Can you work these out from the model? Positions are in its coordinate system, mm. Coordinates: 2 decimals unless noted, no trailing zeros. Order: outer loops, then holes, each group sorted by start corner. A loop starts at its lowest first (then second) coordinate and runs counter-clockwise, first axis right, second up. Notation, with made-up numbers: (-13.5, -31) -> (25.5, -31) arc R20 cw to (25.5, 0) -> close; hole circle Ø2 at (-21.5, 15). An arc over 180 degrees is marked (long way). Return JSON: item names as keys, results as strings. Group by question number.
1) If we section it at D-D, the plane x = 173.5: Please give me the cut outline in (y, z).
2) For pin 1 (6 mm diameter, centred on x = 115.5, y = 11.5, fed in from -Z); pin 2 (6 mm diameter, centred on x = 65.5, y = 11, fed in from +Z); pin 3 (1.8 mm diameter, centred on x = 36.5, z = 20, fed in from +Y), each with a flat end and sliding along its axis, tell me the tip position at first contact or that it passes through.
3) If we section it at B-B, the plane y = 9.5: State how many separate pieces and enclosed holes the cut face has, then the cut area to 3 significant figures.
4) If I drill on probe 1 along Z at (x, y) = (42, 9); probe 2 along X at (y, z) = (4.75, 10) (3 decimals); probe 3 along X at (y, z) = (1.8, 0) (3 decimals), over which ranges is the centre line in solid material (lowest first)? Write a range as from..to.
5) If we section it at A-A, the plane x = 132: Please give me the cut outline in (y, z), then the cut area to 3 significant figures.
6) If we section it at C-C, the plane z = 37.5: Please give me the cut outline in (x, y) (3 decimals), then the cut area to 3 significant figures.
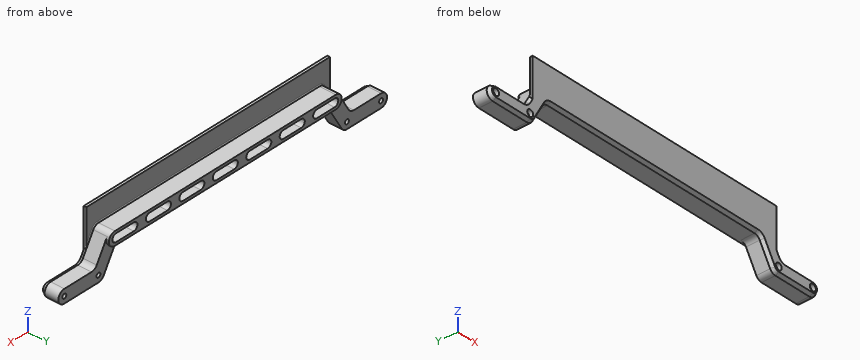
from build123d import *

# Parameters (mm, degrees)
SKETCH_1_R                 = 1.65
EXTRUDE_1_DEPTH            = 15
FILLET_1_R                 = 5
CHAMFER_1_SIZE             = 1.5
CHAMFER_1_SIZE2            = 2.598076211
SKETCH_3_R                 = 2.5
CUT_EXTRUDE_1_DEPTH        = 3
SKETCH_4_W                 = 353.760068279
SKETCH_4_H                 = 71.916373997
CUT_EXTRUDE_2_DEPTH        = 2
FILLET_2_R                 = 5
CUT_EXTRUDE_3_DEPTH        = 12
PATTERN_LINEAR_1_COUNT     = 4
PATTERN_LINEAR_1_PITCH     = 28
PATTERN_LINEAR_1_COL_COUNT = 4
PATTERN_LINEAR_1_COL_PITCH = 28
EXTRUDE_2_DEPTH            = 2
FILLET_3_R                 = 1


# Some blends are built 0.0001 mm under size
with BuildPart() as part:
    # 草图1 → 凸台-拉伸1 (new body)
    with BuildSketch(Plane(origin=(0, 0, 0), x_dir=(1, 0, 0), z_dir=(0, 1, 0))):
        with BuildLine():
            Line((14.275, 5), (-14.275, 5))
            ThreePointArc((-14.275, 5), (-19.275, 0), (-14.275, -5))
            Line((-14.275, -5), (11.388248654, -5))
            Line((11.388248654, -5), (21.491878365, -22.5))
            ThreePointArc((21.491878365, -22.5), (23.322005384, -24.330127019), (25.822005384, -25))
            Line((25.822005384, -25), (210.627994616, -25))
            ThreePointArc((210.627994616, -25), (213.127994616, -24.330127019), (214.958121635, -22.5))
            Line((214.958121635, -22.5), (225.061751346, -5))
            Line((225.061751346, -5), (250.725, -5))
            ThreePointArc((250.725, -5), (255.725, 0), (250.725, 5))
            Line((250.725, 5), (222.175, 5))
            ThreePointArc((222.175, 5), (219.675, 4.330127019), (217.844872981, 2.5))
            Line((217.844872981, 2.5), (207.74124327, -15))
            Line((207.74124327, -15), (28.70875673, -15))
            Line((28.70875673, -15), (18.605127019, 2.5))
            ThreePointArc((18.605127019, 2.5), (16.775, 4.330127019), (14.275, 5))
        make_face()
        with Locations(Location((-14.275, 0, 0), (0, 0, 270))):
            Circle(SKETCH_1_R, mode=Mode.SUBTRACT)
        with Locations(Location((14.275, 0, 0), (0, 0, 270))):
            Circle(SKETCH_1_R, mode=Mode.SUBTRACT)
        with Locations(Location((222.175, 0, 0), (0, 0, 270))):
            Circle(SKETCH_1_R, mode=Mode.SUBTRACT)
        with Locations(Location((250.725, 0, 0), (0, 0, 270))):
            Circle(SKETCH_1_R, mode=Mode.SUBTRACT)
    extrude(amount=EXTRUDE_1_DEPTH)

    # 圆角1
    fillet_1_edges = [part.edges().sort_by_distance(p)[0] for p in [
        (225.061751346, 7.5, 5),
        (11.388248654, 7.5, 5),
        (28.70875673, 7.5, 15),
        (207.74124327, 7.5, 15),
    ]]
    fillet(fillet_1_edges, radius=FILLET_1_R)

    # 倒角1
    chamfer_1_edges = [part.edges().sort_by_distance(p)[0] for p in [
        (255.725, 0, 0),
        (219.288248654, 0, 15),
        (213.127994616, 0, 24.330127019),
        (118.225, 0, 25),
        (23.322005384, 0, 24.330127019),
        (-2.886751346, 0, 5),
        (-19.275, 0, 0),
        (0, 0, -5),
        (16.775, 0, -4.330127019),
        (22.935254038, 0, 5),
        (219.675, 0, -4.330127019),
        (236.45, 0, -5),
        (118.225, 0, 15),
        (213.514745962, 0, 5),
        (239.336751346, 0, 5),
        (17.161751346, 0, 15),
        (207.354491924, 0, 14.330127019),
        (29.095508076, 0, 14.330127019),
        (225.448502692, 0, 5.669872981),
        (11.001497308, 0, 5.669872981),
    ]]
    chamfer_1_side = [part.faces().sort_by_distance(p)[0] for p in [
        (216.892549382, 0, 13.616842381),
    ]]
    chamfer(chamfer_1_edges, length=CHAMFER_1_SIZE, length2=CHAMFER_1_SIZE2, reference=chamfer_1_side[0])

    # 草图3 → 切除-拉伸1 (cut)
    with BuildSketch(Plane(origin=(0, 0, 0), x_dir=(1, 0, 0), z_dir=(0, 1, 0))):
        with Locations(Location((-14.275, 0, 0), (0, 0, 270))):
            Circle(SKETCH_3_R)
        with Locations(Location((14.275, 0, 0), (0, 0, 270))):
            Circle(SKETCH_3_R)
        with Locations(Location((250.725, 0, 0), (0, 0, 270))):
            Circle(SKETCH_3_R)
        with Locations(Location((222.175, 0, 0), (0, 0, 270))):
            Circle(SKETCH_3_R)
    extrude(amount=CUT_EXTRUDE_1_DEPTH, mode=Mode.SUBTRACT)

    # 草图4 → 切除-拉伸2 (cut)
    with BuildSketch(Plane(origin=(0, 15, 0), x_dir=(1, 0, 0), z_dir=(0, 1, 0))):
        with Locations((127.300161481, 20.958186999)):
            Rectangle(SKETCH_4_W, SKETCH_4_H)
    extrude(amount=-CUT_EXTRUDE_2_DEPTH, mode=Mode.SUBTRACT)

    # 圆角2
    fillet_2_edges = [part.edges().sort_by_distance(p)[0] for p in [
        (17.161751346, 14, 15),
        (219.288248654, 14, 15),
    ]]
    fillet(fillet_2_edges, radius=FILLET_2_R - 0.0001)  # a hair under: the kernel refuses the full size

    # 草图5 → 切除-拉伸3 (cut)
    with BuildSketch(Plane(origin=(0, 15, 0), x_dir=(1, 0, 0), z_dir=(0, 1, 0))):
        with BuildLine():
            Line((110.725, -17), (125.725, -17))
            ThreePointArc((125.725, -17), (128.725, -20), (125.725, -23))
            Line((125.725, -23), (110.725, -23))
            ThreePointArc((110.725, -23), (107.725, -20), (110.725, -17))
        make_face()
    cut_extrude_3 = extrude(amount=-CUT_EXTRUDE_3_DEPTH, mode=Mode.SUBTRACT)

    # 阵列(线性)1: 切除-拉伸3 ×4
    with Locations(*[(i * PATTERN_LINEAR_1_PITCH, 0, 0) for i in range(1, PATTERN_LINEAR_1_COUNT)]):
        add(cut_extrude_3, mode=Mode.SUBTRACT)

    # 阵列(线性)1 col: 切除-拉伸3 ×4
    with Locations(*[(-i * PATTERN_LINEAR_1_COL_PITCH, 0, 0) for i in range(1, PATTERN_LINEAR_1_COL_COUNT)]):
        add(cut_extrude_3, mode=Mode.SUBTRACT)

    # 草图6 → 凸台-拉伸2 (add)
    with BuildSketch(Plane.XZ):
        Polygon((25.533330249, 23.5), (210.339319482, 23.5), (220.175, 6.464101615), (220.175, 23.5), (220.175, 40), (16.275, 40), (16.275, 23), (16.275, 7.464101615), align=None)
    extrude(amount=-EXTRUDE_2_DEPTH)

    # 圆角3
    # the kernel refuses this fillet: 1 mm, written as the material it adds along each edge
    with BuildSketch(Plane(origin=(214.659083529, 2, 22.327350269), x_dir=(0.4330127018948014, 0.8660254037827173, 0.2500000000014904), z_dir=(0.4999999999999995, 0, -0.866025403784439))) as fillet_3_piece_1_section:
        with BuildLine():
            CenterArc((1.496511696, 0.592034292), FILLET_3_R, 150, 66.301500994)
            Line((0.630486292, 1.092034292), (0.613165784, 1.102034292))
            Line((0.613165784, 1.102034292), (-0.017320508, 0.01))
            Line((-0.017320508, 0.01), (0, -0.02))
            ThreePointArc((0, -0.02), (0.345299462, -0.02), (0.674480668, -0.011840686))
            Line((0.674480668, -0.011840686), (0.690598923, 0))
        make_face()
    fillet_3_piece_1 = extrude(amount=14.184264403, mode=Mode.PRIVATE)
    fillet_3_piece_1 = split(fillet_3_piece_1, bisect_by=Plane(origin=(220.175, 2.148183279, 18.272519996), z_dir=(-1, 0, 0)), keep=Keep.TOP, mode=Mode.PRIVATE)
    add(fillet_3_piece_1)
    with BuildSketch(Plane(origin=(210.627994616, 2, 20), x_dir=(0, 0, 1), z_dir=(-1, 0, 0))) as fillet_3_piece_2:
        with BuildLine():
            CenterArc((5.915673123, 1), FILLET_3_R, 203.698499006, 66.301500994)
            Line((5.915673123, 0), (5.915673123, -0.02))
            Line((5.915673123, -0.02), (4.654700538, -0.02))
            Line((4.654700538, -0.02), (4.63738003, 0.01))
            ThreePointArc((4.63738003, 0.01), (4.810029761, 0.309038106), (4.981686538, 0.590037736))
            Line((4.981686538, 0.590037736), (5, 0.598076211))
        make_face()
    revolve(axis=Axis((210.627994616, 2, 20), (0, 1, 0)), revolution_arc=60)
    with BuildSketch(Plane(origin=(25.822005384, 2, 24.654700538), x_dir=(0, 0, 1), z_dir=(1, 0, 0))) as fillet_3_piece_3:
        with BuildLine():
            CenterArc((1.260972585, -1), FILLET_3_R, 90, 66.301500994)
            Line((0.345299462, -0.598076211), (0.326985999, -0.590037736))
            ThreePointArc((0.326985999, -0.590037736), (0.155329223, -0.309038106), (-0.017320508, -0.01))
            Line((-0.017320508, -0.01), (0, 0.02))
            Line((0, 0.02), (1.260972585, 0.02))
            Line((1.260972585, 0.02), (1.260972585, 0))
        make_face()
    extrude(amount=184.805989232)
    with BuildSketch(Plane(origin=(25.822005384, 2, 20), x_dir=(-0.8660254037844389, 0, 0.49999999999999944), z_dir=(-0.49999999999999944, 0, -0.8660254037844389))) as fillet_3_piece_4:
        with BuildLine():
            CenterArc((5.915673123, 1), FILLET_3_R, 203.698499006, 66.301500994)
            Line((5, 0.598076211), (4.981686538, 0.590037736))
            ThreePointArc((4.981686538, 0.590037736), (4.810029761, 0.309038106), (4.63738003, 0.01))
            Line((4.63738003, 0.01), (4.654700538, -0.02))
            Line((4.654700538, -0.02), (5.915673123, -0.02))
            Line((5.915673123, -0.02), (5.915673123, 0))
        make_face()
    revolve(axis=Axis((25.822005384, 2, 20), (0, 1, 0)), revolution_arc=60)
    with BuildSketch(Plane(origin=(14.698784269, 2, 10.043416963), x_dir=(-0.86602540378444, 0, 0.4999999999999978), z_dir=(0.4999999999999977, 0, 0.86602540378444))) as fillet_3_piece_5_section:
        with BuildLine():
            CenterArc((1.260972585, -1), FILLET_3_R, 90, 66.301500994)
            Line((0.345299462, -0.598076211), (0.326985999, -0.590037736))
            ThreePointArc((0.326985999, -0.590037736), (0.155329223, -0.309038106), (-0.017320508, -0.01))
            Line((-0.017320508, -0.01), (0, 0.02))
            Line((0, 0.02), (1.260972585, 0.02))
            Line((1.260972585, 0.02), (1.260972585, 0))
        make_face()
    fillet_3_piece_5 = extrude(amount=14.184264403, mode=Mode.PRIVATE)
    fillet_3_piece_5 = split(fillet_3_piece_5, bisect_by=Plane(origin=(16.275, 2.148183279, 18.272519996), z_dir=(1, 0, 0)), keep=Keep.TOP, mode=Mode.PRIVATE)
    add(fillet_3_piece_5)


solid = part.part
Result sheet:
{
 "1": {"outline": "(0, 16.5) -> (2.6, 15) -> (15, 15) -> (15, 17) -> (3, 17) -> (3, 23) -> (15, 23) -> (15, 25) -> (2.6, 25) arc R1 cw to (2, 25.92) -> (2, 40) -> (0, 40) -> close"},
 "2": {"pin 1": "stops at z = 15", "pin 2": "stops at z = 25", "pin 3": "stops at y = 3"},
 "3": {"separate pieces": "1", "enclosed holes": "11", "area": "2,100 mm2"},
 "4": {"probe 1": "z = 15..17.01, 22.99..25", "probe 2": "x = 14.275..25.822, 210.628..222.175", "probe 3": "x = -18.814..-16.775, -11.775..11.775, 16.775..19.516, 216.934..219.675, 224.675..248.225, 253.225..255.264"},
 "5": {"outline": "(0, 16.5) -> (2.6, 15) -> (15, 15) -> (15, 25) -> (2.6, 25) arc R1 cw to (2, 25.92) -> (2, 40) -> (0, 40) -> close", "area": "178 mm2"},
 "6": {"outline": "(16.275, 0) -> (220.175, 0) -> (220.175, 2) -> (16.275, 2) -> close", "area": "408 mm2"}
}
